Geometry check sheet. Reference: the model listing, model coordinates, mm. A direction names the side the tool comes from. Round coordinates to 2 decimals unless told otherwise and drop trailing zeros. Write each loop counter-clockwise with the first axis right and the second up, starting at its lowest first coordinate (ties: lowest second). Pieces come first, ordered by that corner, then holes. Notation, with made-up numbers: M -21,49.25 L 6,49.25 A28 cw 6,70.25 Z; hole C 43,86 d6. An arc over 180 degrees is marked long. Use a Markdown table: item, result.
Autodesk Fusion 360 part; units mm, degrees
sketch "Sketch1" plane through (0, 0, 0) normal (0, 1, 0) x (1, 0, 0)
  line L0 (85, -20) -> (-85, -20)
  line L1 (-85, -20) -> (-85, 20)
  line L2 (-85, 20) -> (85, 20)
  line L3 (85, 20) -> (85, -20)
  circle A0 centre (0, 0) radius 14
  line L4 (71.9, 10) -> (71.9, -10)
  arc A1 (71.9, -10) -> (78.1, -10) centre (75, -10) ccw
  line L5 (78.1, -10) -> (78.1, 10)
  arc A2 (78.1, 10) -> (71.9, 10) centre (75, 10) ccw
  line L6 (-71.9, 10) -> (-71.9, -10)
  arc A3 (-71.9, 10) -> (-78.1, 10) centre (-75, 10) ccw
  line L7 (-78.1, -10) -> (-78.1, 10)
  arc A4 (-78.1, -10) -> (-71.9, -10) centre (-75, -10) ccw
  dimension "d1" = 170
  dimension "d2" = 40
  dimension "d4" = 28
  dimension "d7" = 20
  dimension "d10" = 6.2
  dimension "d11" = 150
extrude "Extrude1" add sketch "Sketch1" along normal blind 4
Item 1: Mould release check, pull along Z, two halves, no side actions. Record for faces 3 (the face through (-1, 0, 17)), 4 (the face through (1, 2, 20)), 5 (the face through (74.9, 2, -13.1)): +Z half, -Z half, draft (parallel to the pull), parting line (faces both ways), or undercut.
Outcome:
| item | result |
|---|---|
| face 3 | draft |
| face 4 | +Z half |
| face 5 | undercut |
Item 2: Access from +Z, -Z, +X, -X, +Y, -Y to the whole of each face (thin tool, end or side, straight path). Record for faces 1 (the face through (-85, 2, 0)), 2 (the face through (-78.1, 2, 0)).
Outcome:
| item | result |
|---|---|
| face 1 | +Z, -Z, -X, +Y, -Y |
| face 2 | +Y, -Y |
Item 3: Cross-section at A-A, the plane z = 0. Record the cut outline in (x, y), and give its area (3 significant figures).
Outcome:
| item | result |
|---|---|
| outline | M -85,0 L -78.1,0 L -78.1,4 L -85,4 Z; M -71.9,0 L -14,0 L -14,4 L -71.9,4 Z; M 14,0 L 71.9,0 L 71.9,4 L 14,4 Z; M 78.1,0 L 85,0 L 85,4 L 78.1,4 Z |
| area | 518 mm2 |
Item 4: Material ranges on line 1 along X through (y, z) = (0.85, 0); line 2 along Z through (x, y) = (0, 1.95); line 3 along X through (y, z) = (2.4, 1.5), recorded low to high. Write a range as from..to.
Outcome:
| item | result |
|---|---|
| line 1 | x = -85..-78.1, -71.9..-14, 14..71.9, 78.1..85 |
| line 2 | z = -20..-14, 14..20 |
| line 3 | x = -85..-78.1, -71.9..-13.92, 13.92..71.9, 78.1..85 |
Item 5: Cross-section at D-D, the plane x = -75. Record the cut outline in (y, z), and give its area (3 significant figures).
Outcome:
| item | result |
|---|---|
| outline | M 0,-20 L 4,-20 L 4,-13.1 L 0,-13.1 Z; M 0,13.1 L 4,13.1 L 4,20 L 0,20 Z |
| area | 55.2 mm2 |
Item 6: Cross-section at C-C, the plane y = 1.3. Record the cut outline in (x, z), and give its area (3 significant figures).
Outcome:
| item | result |
|---|---|
| outline | M -85,-20 L 85,-20 L 85,20 L -85,20 Z; hole M -78.1,-10 A3.1 ccw -71.9,-10 L -71.9,10 A3.1 ccw -78.1,10 Z; hole C 0,0 d28; hole M 71.9,-10 A3.1 ccw 78.1,-10 L 78.1,10 A3.1 ccw 71.9,10 Z |
| area | 5,880 mm2 |
Item 7: Cross-section at B-B, the plane x = 0. Record the cut outline in (y, z), and give its area (3 significant figures).
Outcome:
| item | result |
|---|---|
| outline | M 0,-20 L 4,-20 L 4,-14 L 0,-14 Z; M 0,14 L 4,14 L 4,20 L 0,20 Z |
| area | 48.0 mm2 |
